Autodesk Inventor part; units mm, degrees
ref_plane "YZ Plane" through (0, 0, 0) normal (1, 0, 0) x (0, 1, 0)
ref_plane "XZ Plane" through (0, 0, 0) normal (0, 1, 0) x (-1, 0, 0)
ref_plane "XY Plane" through (0, 0, 0) normal (0, 0, 1) x (1, 0, 0)
sketch "Sketch1" plane through (0, 0, 0) normal (1, 0, 0) x (0, 1, 0)
  line L0 (0, 0) -> (406.4, 0)
  line L1 (406.4, 0) -> (406.4, -406.4)
  line L2 (406.4, -406.4) -> (0, -406.4)
  line L3 (0, -406.4) -> (0, 0)
  dimension "d0" = 406.4
  dimension "d1" = 406.4
extrude "Extrusion1" add sketch "Sketch1" along normal blind 12.7
sketch "Sketch2" plane through (12.7, 0, 0) normal (1, 0, 0) x (0, 0, -1)
  arc A0 (253.151, 217.4875) -> (253.151, 188.9125) centre (133.35, 203.2) ccw
  arc A1 (278.9512, 188.9125) -> (278.9512, 217.4875) centre (327.7007, 203.2) ccw
  line L0 (0, 406.4) -> (0, 0)
  line L1 (406.4, 406.4) -> (0, 406.4)
  line L2 (327.7007, 203.2) -> (213.4007, 203.2) construction
  line L3 (327.7007, 217.4875) -> (213.4007, 217.4875)
  line L4 (213.4007, 188.9125) -> (327.7007, 188.9125)
  arc A2 (327.7007, 188.9125) -> (327.7007, 217.4875) centre (327.7007, 203.2) ccw
  arc A3 (213.4007, 217.4875) -> (213.4007, 188.9125) centre (213.4007, 203.2) ccw
  point P0 (270.5507, 203.2)
  dimension "d4" = 241.3
  dimension "d5" = 101.6
  dimension "d6" = 133.35
  dimension "d7" = 12.7
  dimension "d8" = 203.2
  dimension "d9" = 203.2
  dimension "d10" = 114.3
  dimension "d11" = 28.575
extrude "Extrusion2" cut sketch "Sketch2" against normal blind 25.4 contours L3 A2 L4 A3
properties part number "Prototype Panel2"
Here's how the part is built. I have some questions about the finished solid (model axes, mm). A direction names the side the tool comes from. Round coordinates to 2 decimals unless told otherwise and drop trailing zeros. Loops run counter-clockwise (first coordinate to the right, second up) from the corner with the lowest first, then second, coordinate; pieces in that order, holes last.
1. If I drill on line 1 along Y through (x, z) = (3.25, -312.5), over which ranges is the centre line in solid material (lowest first)?
Answer list:
line 1: y = 0 to 188.91, 217.49 to 406.4
2. We'd pull the mould along Y, two halves only. Please class faces 3 (the face through (6, 406.4, -200)), 4 (the face through (0, 200, -155)), 5 (the face through (6, 217.488, -271)): +Y half, -Y half, draft (parallel to the pull), parting line (faces both ways), or undercut.
Answer list:
face 3: +Y half
face 4: draft
face 5: undercut
3. Which directions (+Z, -Z, +X, -X, +Y, -Y) give clear straight access to the entire face, cutting with the end or side of a thin tool? Please do faces 1 (the face through (6, 0, -206)), 2 (the face through (6, 188.912, -270)).
Answer list:
face 1: +Z, -Z, +X, -X, -Y
face 2: +X, -X
4. If we section it at B-B on z = -282: Write out the boundary of the cut face in (x, y).
Answer list:
outline: (0, 0) - (12.7, 0) - (12.7, 188.91) - (0, 188.91) - close; (0, 217.49) - (12.7, 217.49) - (12.7, 406.4) - (0, 406.4) - close
5. If we section it at A-A on y = 203.2: Write out the boundary of the cut face in (x, z).
Answer list:
outline: (0, -406.4) - (12.7, -406.4) - (12.7, -341.99) - (0, -341.99) - close; (0, -199.11) - (12.7, -199.11) - (12.7, 0) - (0, 0) - close
6. If we section it at C-C on x = 10: Write out the boundary of the cut face in (y, z) (1 decimal).
Answer list:
outline: (0, -406.4) - (406.4, -406.4) - (406.4, 0) - (0, 0) - close; hole (188.9, -327.7) arc R14.3 ccw to (217.5, -327.7) - (217.5, -213.4) arc R14.3 ccw to (188.9, -213.4) - close
